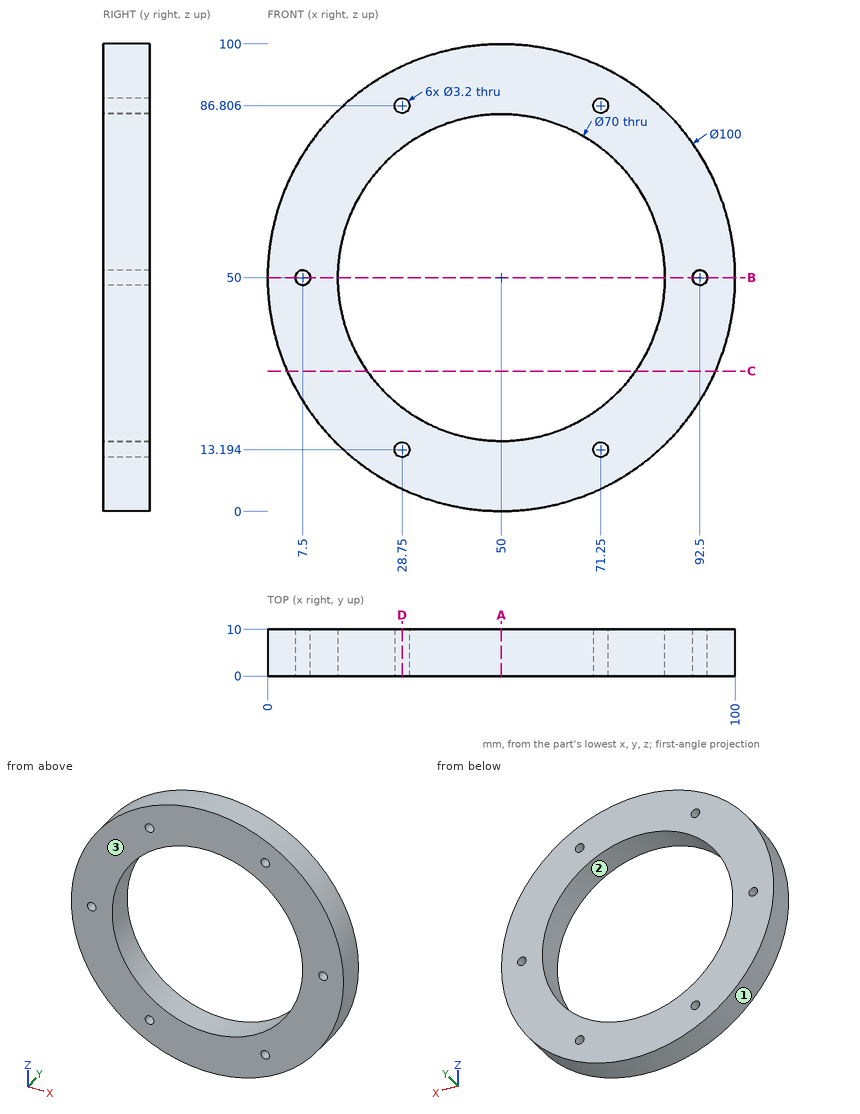
For this review, use the dimensioned drawing (mm, ordinates from the lowest corner) and the shaded views. Give positions to 0.01 mm unless a question says otherwise; leave off trailing zeros. Write each loop counter-clockwise with the first axis right and the second up, starting at its lowest first coordinate (ties: lowest second). Pieces come first, ordered by that corner, then holes. Notation, with made-up numbers: M -31,31.5 L -2,31.5 A18 cw -2,57.5 Z; hole C 25,-21.5 d11. An arc over 180 degrees is marked long. Answer as a JSON object with one key per item and string values. Group by question number.
1) We need section B-B (z = 50). Give the boundary of the cut face in (x, y), and give its area (3 significant figures).
2) Clearance check with flat-ended pins moving along their axes: pin 1 Ø2 at (x, y) = (84, 8.5) entering from +Z; pin 2 Ø1 at (x, y) = (37.5, 3) entering from -Z; pin 3 Ø1.9 at (x, z) = (92.5, 50) entering from +Y; pin 4 Ø4 at (x, y) = (40.5, 7.5) entering from -Z. State where each tip first meets the part, or that it passes through.
3) We need section D-D (x = 28.75). Give the boundary of the cut face in (y, z).
4) We need section C-C (z = 30). Give the boundary of the cut face in (x, y), and give its area (3 significant figures).
5) Mouldability with a two-part tool opening along X and no side actions: class the marked faces 1, 2 and 3 as released by +X, released by -X, zero draft, split by the parting line, or undercut.
6) We need section A-A (x = 50). Give the boundary of the cut face in (y, z).
7) For line 1 along X through (y, z) = (7.5, 50); line 2 along Z through (x, y) = (22.5, 9.25); line 3 along X through (y, z) = (4, 86.5), list the stretches that pass through material, from the lowest coordinate up.
Answer key:
{
 "1": {"outline": "M 0,0 L 5.9,0 L 5.9,10 L 0,10 Z; M 9.1,0 L 15,0 L 15,10 L 9.1,10 Z; M 85,0 L 90.9,0 L 90.9,10 L 85,10 Z; M 94.1,0 L 100,0 L 100,10 L 94.1,10 Z", "area": "236 mm²"},
 "2": {"pin 1": "stops at z = 87.56", "pin 2": "stops at z = 1.46", "pin 3": "passes through", "pin 4": "stops at z = 0.57"},
 "3": {"outline": "M 0,4.74 L 10,4.74 L 10,11.59 L 0,11.59 Z; M 0,14.79 L 10,14.79 L 10,22.19 L 0,22.19 Z; M 0,77.81 L 10,77.81 L 10,85.21 L 0,85.21 Z; M 0,88.41 L 10,88.41 L 10,95.26 L 0,95.26 Z"},
 "4": {"outline": "M 4.17,0 L 21.28,0 L 21.28,10 L 4.17,10 Z; M 78.72,0 L 95.83,0 L 95.83,10 L 78.72,10 Z", "area": "342 mm²"},
 "5": {"face 1": "split by the parting line", "face 2": "undercut", "face 3": "zero draft"},
 "6": {"outline": "M 0,0 L 10,0 L 10,15 L 0,15 Z; M 0,85 L 10,85 L 10,100 L 0,100 Z"},
 "7": {"line 1": "x = 0 to 5.9, 9.1 to 15, 85 to 90.9, 94.1 to 100", "line 2": "z = 8.24 to 28.35, 71.65 to 91.76", "line 3": "x = 15.83 to 27.18, 30.32 to 69.68, 72.82 to 84.17"}
}
